from build123d import *


with BuildPart() as part:
    # Sketch1 → Revolve1 (revolve)
    with BuildSketch(Plane.XY):
        Polygon((-82.105117767, 11.5), (0, 33.5), (0, 38.5), (-76.4, 18.028681698), (-76.4, 44.496311912), (-96.4, 44.496311912), (-96.4, 41.496311912), (-101.4, 41.496311912), (-101.4, 44.496311912), (-106.4, 44.496311912), (-106.4, 41.496311912), (-111.4, 41.496311912), (-111.4, 44.496311912), (-116.4, 44.496311912), (-116.4, 41.496311912), (-121.4, 41.496311912), (-121.4, 44.496311912), (-126.4, 44.496311912), (-126.4, 36.496311912), (-83.105117767, 11.5), align=None)
    revolve(axis=Axis((0, 0, 0), (-1, 0, 0)))

    # Sketch2 → Cut-Revolve1 (revolve, cut)
    with BuildSketch(Plane.XY):
        Polygon((-11.196152423, 0), (-11.196152423, 35.5), (-11.196152423, 56.271944123), (14.531335426, 56.271944123), (14.531335426, 0), align=None)
    revolve(axis=Axis((0, 0, 0), (-1, 0, 0)), mode=Mode.SUBTRACT)


solid = part.part
Geometry check sheet. Reference: the model listing, model coordinates, mm. A direction names the side the tool comes from. Coordinates: 2 decimals unless noted, no trailing zeros. Order: outer loops, then holes, each group sorted by start corner. A loop starts at its lowest first (then second) coordinate and runs counter-clockwise, first axis right, second up. Notation, with made-up numbers: (-18, -26) - (35, -26) arc R23 cw to (35, 10) - close; hole circle Ø11 at (-36.75, -3). An arc over 180 degrees is marked (long way). Answer in a Markdown table with one row per item. Add a question column.
1) Cross-section at B-B, the plane x = -95. Record the cut outline in (y, z), then the cut area to 3 significant figures.
2) Material ranges on line 1 along Z through (x, y) = (-82.6, 0); line 2 along Y through (x, z) = (-82, 0); line 3 along X through (y, z) = (25, 35), recorded low to high. Write a range as [from, to].
3) Release check for a two-part mould opening along X. For faces 3 (the cylindrical face through (-103.94, -5.79, -44.12)), 4 (the flat face through (-11.196, 15.6, -26.5)), 5 (the flat face through (-116.4, 29.5, 29.5)) record: +X half, -X half, draft (parallel to the pull), parting line (faces both ways), or undercut.
4) Cross-section at A-A, the plane x = -48. Record the cut outline in (y, z).
5) Gauge pin test, flat ends, axial feed: P1, Ø8, axis at x = -57, z = 17, coming from the +Y side; P2, Ø8, axis at x = -41.5, z = 19.5, coming from the +Y side; P3, Ø1, axis at x = -67.5, y = -14, coming from the -Z side. Record the tip position at first contact, or that the pin passes through.
6) Set-up check for faces 1 (the flat face through (-101.4, -29.5, 29.5)), 2 (the cylindrical face through (-123.94, -5.79, -44.12)): record each of +Z, -Z, +X, -X, +Y, -Y from which the full face is reachable in a straight line by a thin tool's end or side.
Check result:
| question | item | result |
|---|---|---|
| 1 | outline | circle Ø88.99 at (0, 0); hole circle Ø36.74 at (0, 0) |
| 1 | area | 5,160 mm² |
| 2 | line 1 | z = [-44.5, -11.5], [11.5, 44.5] |
| 2 | line 2 | y = [-44.5, -11.53], [11.53, 44.5] |
| 2 | line 3 | x = [-126.4, -121.4], [-116.4, -111.4], [-106.4, -101.4], [-96.4, -76.4] |
| 3 | face 3 | draft |
| 3 | face 4 | +X half |
| 3 | face 5 | undercut |
| 4 | outline | circle Ø51.28 at (0, 0); hole circle Ø41.28 at (0, 0) |
| 5 | P1 | stops at y = 19.54 |
| 5 | P2 | stops at y = 22.86 |
| 5 | P3 | stops at z = -15.35 |
| 6 | face 1 | none |
| 6 | face 2 | +X, -X |
